from build123d import *

# Parameters (mm, degrees)
F0_W     = 116.443158
F0_H     = 48.552304
F1_DEPTH = 30
F2_SIZE  = 20
F3_SIZE  = 20


with BuildPart() as f1:
    # F0 (on Front) → F1 (new body)
    with BuildSketch(Plane.XZ):
        Rectangle(F0_W, F0_H)
    extrude(amount=F1_DEPTH)

    # F2
    f2_edges = [f1.edges().sort_by_distance(p)[0] for p in [
        (0, -30, 24.276152),
    ]]
    chamfer(f2_edges, length=F2_SIZE)

    # F3
    f3_edges = [f1.edges().sort_by_distance(p)[0] for p in [
        (-58.221579, -30, -10),
        (58.221579, -30, -10),
    ]]
    chamfer(f3_edges, length=F3_SIZE)


solid = f1.part
Source: CAD feature listing. Evaluate the final solid. Frame: model axes, mm. Round coordinates to 2 decimals unless told otherwise and drop trailing zeros. Loops run counter-clockwise (first coordinate to the right, second up) from the corner with the lowest first, then second, coordinate; pieces in that order, holes last. Notation, with made-up numbers: (-35, 55.25) -> (3, 55.25) arc R21 cw to (3, 84.25) -> close; hole circle Ø8 at (25, -27.5). An arc over 180 degrees is marked (long way). Answer as a JSON object with one key per item and string values. Group by question number.
Q1. Contact query for flat-ended pins moving along their axis: P1, Ø12, axis at y = -18.5, z = -8, coming from the -X side; P2, Ø8, axis at x = 25.5, y = -27, coming from the +Z side. Output: stop coordinate, or through.
Q2. Section query A-A (z = -13.5). Output: boundary loops of the cut face in (x, y), plus the area to 3 significant figures.
Q3. Section query B-B (x = -4). Output: boundary loops of the cut face in (y, z), plus the area to 3 significant figures.
Q4. Ray query, line 1 (Z direction, x = -19, y = -28); line 2 (Y direction, x = 51.5, z = -20); line 3 (X direction, y = -14, z = 19). Return the intervals inside material, ascending. Write a range as from..to.
Q5. Section query D-D (x = 48). Output: boundary loops of the cut face in (y, z).
Q6. Section query C-C (y = -15.5). Output: boundary loops of the cut face in (x, z).
Completed:
{
 "1": {"P1": "x = -55.72", "P2": "z = 11.28"},
 "2": {"outline": "(-58.22, -10) -> (-38.22, -30) -> (38.22, -30) -> (58.22, -10) -> (58.22, 0) -> (-58.22, 0) -> close", "area": "3,090 mm²"},
 "3": {"outline": "(-30, -24.28) -> (0, -24.28) -> (0, 24.28) -> (-10, 24.28) -> (-30, 4.28) -> close", "area": "1,260 mm²"},
 "4": {"line 1": "-24.28..6.28", "line 2": "-16.72..0", "line 3": "-54.22..54.22"},
 "5": {"outline": "(-20.22, -24.28) -> (0, -24.28) -> (0, 24.28) -> (-10, 24.28) -> (-20.22, 14.05) -> close"},
 "6": {"outline": "(-52.72, -24.28) -> (52.72, -24.28) -> (52.72, 18.78) -> (-52.72, 18.78) -> close"}
}
